```python
from build123d import *

# Parameters (mm, degrees)
SKETCH_R        = 1.75
PAD_DEPTH       = 2
PAD001_DEPTH    = 13
SKETCH002_W     = 76.2
SKETCH002_H     = 61.2
PAD002_DEPTH    = 2
PAD003_DEPTH    = 25
SKETCH004_W     = 14.2
SKETCH004_H     = 19
SKETCH004_W_2   = 29
POCKET_DEPTH    = 2
SKETCH005_W     = 66.2
SKETCH005_H     = 19
POCKET001_DEPTH = 2
SKETCH006_W     = 35
SKETCH006_H     = 25
SKETCH006_W_2   = 14.2
SKETCH006_H_2   = 19
POCKET002_DEPTH = 2
PAD004_DEPTH    = 2
PAD005_DEPTH    = 26
SKETCH009_W     = 51.2
SKETCH009_H     = 20
POCKET003_DEPTH = 2
SKETCH010_W     = 66.2
SKETCH010_H     = 20
POCKET004_DEPTH = 2
SKETCH011_W     = 51.2
SKETCH011_H     = 20
POCKET005_DEPTH = 2
PAD006_DEPTH    = 2
SKETCH013_W     = 5
SKETCH013_H     = 3
PAD007_DEPTH    = 2
SKETCH014_W     = 6
SKETCH014_H     = 6
SKETCH014_R     = 1.25
PAD008_DEPTH    = 6
SKETCH015_W     = 8
SKETCH015_H     = 20
POCKET006_DEPTH = 5
SKETCH016_W     = 20
SKETCH016_H     = 24
POCKET007_DEPTH = 5


with BuildPart() as part:
    # Sketch → Pad (new body)
    with BuildSketch(Plane.XY):
        Polygon((0, 28.537386), (-24.714102, -14.268693), (24.714102, -14.268693), align=None)
        with Locations((7.160898, 4.134347)):
            Circle(SKETCH_R, mode=Mode.SUBTRACT)
        with Locations((0, -8.268693)):
            Circle(SKETCH_R, mode=Mode.SUBTRACT)
        with Locations((-7.160898, 4.134347)):
            Circle(SKETCH_R, mode=Mode.SUBTRACT)
        Polygon((0, 8.537386), (-7.393594, -4.268693), (7.393594, -4.268693), align=None, mode=Mode.SUBTRACT)
    extrude(amount=PAD_DEPTH)

    # Sketch001 (on Face11 of Pad) → Pad001 (join)
    with BuildSketch(Plane.XY.offset(2)):
        Polygon((0, 28.537386), (-24.714102, -14.268693), (24.714102, -14.268693), align=None)
        Polygon((0, 24.537386), (-21.25, -12.268693), (21.25, -12.268693), align=None, mode=Mode.SUBTRACT)
    extrude(amount=PAD001_DEPTH)

    # Sketch002 (on Face14 of Pad001) → Pad002 (join)
    with BuildSketch(Plane.XY.offset(15)):
        with Locations((0, 1.4)):
            Rectangle(SKETCH002_W, SKETCH002_H)
        Polygon((0, 24.537386), (-21.25, -12.268693), (21.25, -12.268693), align=None, mode=Mode.SUBTRACT)
    extrude(amount=PAD002_DEPTH)

    # Sketch003 (on Face23 of Pad002) → Pad003 (join)
    with BuildSketch(Plane.XY.offset(17)):
        Polygon((-38.1, -29.2), (-38.1, 32), (38.1, 32), (38.1, -29.2), (36.1, -29.2), (36.1, -7), (28.1, -7), (28.1, -5), (36.1, -5), (36.1, 30), (-36.1, 30), (-36.1, -5), (-28.1, -5), (-28.1, -7), (-36.1, -7), (-36.1, -29.2), align=None)
    extrude(amount=PAD003_DEPTH)

    # Sketch004 (on Face39 of Pad003) → Pocket (cut)
    with BuildSketch(Plane.YZ.offset(-36.1)):
        with Locations((-17.1, 29.5)):
            Rectangle(SKETCH004_W, SKETCH004_H)
        with Locations((12.5, 29.5)):
            Rectangle(SKETCH004_W_2, SKETCH004_H)
    extrude(amount=-POCKET_DEPTH, mode=Mode.SUBTRACT)

    # Sketch005 (on Face46 of Pocket) → Pocket001 (cut)
    with BuildSketch(Plane.XZ.offset(-30)):
        with Locations((0, 29.5)):
            Rectangle(SKETCH005_W, SKETCH005_H)
    extrude(amount=-POCKET001_DEPTH, mode=Mode.SUBTRACT)

    # Sketch006 (on Face49 of Pocket001) → Pocket002 (cut)
    with BuildSketch(Plane(origin=(36.1, 0, 0), x_dir=(0, -1, 0), z_dir=(-1, 0, 0))):
        with Locations((-12.5, 29.5)):
            Rectangle(SKETCH006_W, SKETCH006_H)
        with Locations((17.1, 29.5)):
            Rectangle(SKETCH006_W_2, SKETCH006_H_2)
    extrude(amount=-POCKET002_DEPTH, mode=Mode.SUBTRACT)

    # Sketch007 (on Face34 of Pocket002) → Pad004 (join)
    with BuildSketch(Plane.XY.offset(42)):
        Polygon((-38.1, -29.2), (-38.1, 32), (38.1, 32), (38.1, -29.2), (28.1, -29.2), (28.1, 22), (-28.1, 22), (-28.1, -29.2), align=None)
    extrude(amount=PAD004_DEPTH)

    # Sketch008 (on Face67 of Pad004) → Pad005 (join)
    with BuildSketch(Plane.XY.offset(44)):
        Polygon((-38.1, -29.2), (-38.1, 32), (38.1, 32), (38.1, -29.2), (36.1, -29.2), (36.1, 30), (-36.1, 30), (-36.1, -29.2), align=None)
    extrude(amount=PAD005_DEPTH)

    # Sketch009 (on Face82 of Pad005) → Pocket003 (cut)
    with BuildSketch(Plane.YZ.offset(-36.1)):
        with Locations((1.4, 57)):
            Rectangle(SKETCH009_W, SKETCH009_H)
    extrude(amount=-POCKET003_DEPTH, mode=Mode.SUBTRACT)

    # Sketch010 (on Face85 of Pocket003) → Pocket004 (cut)
    with BuildSketch(Plane.XZ.offset(-30)):
        with Locations((0, 57)):
            Rectangle(SKETCH010_W, SKETCH010_H)
    extrude(amount=-POCKET004_DEPTH, mode=Mode.SUBTRACT)

    # Sketch011 (on Face88 of Pocket004) → Pocket005 (cut)
    with BuildSketch(Plane(origin=(36.1, 0, 0), x_dir=(0, -1, 0), z_dir=(-1, 0, 0))):
        with Locations((-1.4, 57)):
            Rectangle(SKETCH011_W, SKETCH011_H)
    extrude(amount=-POCKET005_DEPTH, mode=Mode.SUBTRACT)

    # Sketch012 (on Face78 of Pocket005) → Pad006 (join)
    with BuildSketch(Plane.XY.offset(70)):
        Polygon((-38.1, -29.2), (-38.1, 32), (38.1, 32), (38.1, -29.2), (31.1, -29.2), (31.1, -25.2), (34.1, -25.2), (34.1, 28), (-34.1, 28), (-34.1, -25.2), (-31.1, -25.2), (-31.1, -29.2), align=None)
    extrude(amount=PAD006_DEPTH)

    # Sketch013 (on Face98 of Pad006) → Pad007 (join)
    with BuildSketch(Plane.XZ.offset(29.2)):
        with Locations((-33.6, 68.5)):
            Rectangle(SKETCH013_W, SKETCH013_H)
        with Locations((33.6, 68.5)):
            Rectangle(SKETCH013_W, SKETCH013_H)
    extrude(amount=-PAD007_DEPTH)

    # Sketch014 (on Face19 of Pad007) → Pad008 (join)
    with BuildSketch(Plane.XZ.offset(29.2)):
        with Locations((31.1, 12)):
            Rectangle(SKETCH014_W, SKETCH014_H)
        with Locations((31.1, 12)):
            Circle(SKETCH014_R, mode=Mode.SUBTRACT)
        with Locations((-8.9, 12)):
            Rectangle(SKETCH014_W, SKETCH014_H)
        with Locations((-8.9, 12)):
            Circle(SKETCH014_R, mode=Mode.SUBTRACT)
    extrude(amount=-PAD008_DEPTH)

    # Sketch015 (on Face83 of Pad008) → Pocket006 (cut)
    with BuildSketch(Plane.XY.offset(44)):
        with Locations((-32.1, 5)):
            Rectangle(SKETCH015_W, SKETCH015_H)
    extrude(amount=-POCKET006_DEPTH, mode=Mode.SUBTRACT)

    # Sketch016 (on Face61 of Pocket006) → Pocket007 (cut)
    with BuildSketch(Plane.YZ.offset(-36.1)):
        with Locations((5, 32)):
            Rectangle(SKETCH016_W, SKETCH016_H)
    extrude(amount=-POCKET007_DEPTH, mode=Mode.SUBTRACT)


solid = part.part
```
Part model, mm, in its own coordinate system. A direction names the side the tool comes from. Round coordinates to 2 decimals unless told otherwise and drop trailing zeros. Loops run counter-clockwise (first coordinate to the right, second up) from the corner with the lowest first, then second, coordinate; pieces in that order, holes last.
1. Slice it at A-A (z = 12). Give the cut face in (x, y).
Solutions:
outline: (-24.71, -14.27) - (24.71, -14.27) - (0, 28.54) - close; (-11.9, -29.2) - (-10.15, -29.2) - (-10.15, -23.2) - (-11.9, -23.2) - close; (-7.65, -29.2) - (-5.9, -29.2) - (-5.9, -23.2) - (-7.65, -23.2) - close; (28.1, -29.2) - (29.85, -29.2) - (29.85, -23.2) - (28.1, -23.2) - close; (32.35, -29.2) - (34.1, -29.2) - (34.1, -23.2) - (32.35, -23.2) - close; hole (-21.25, -12.27) - (21.25, -12.27) - (0, 24.54) - close
2. Slice it at B-B (x = 4). Count the separate pieces of the cut face and the enclosed holes in it, and give its area (3 significant figures).
Solutions:
separate pieces: 4
enclosed holes: 0
area: 253 mm2
3. Slice it at C-C (z = 52). Give the cut face in (x, y).
Solutions:
outline: (-38.1, -29.2) - (-36.1, -29.2) - (-36.1, -24.2) - (-38.1, -24.2) - close; (-38.1, 27) - (-36.1, 27) - (-36.1, 30) - (-33.1, 30) - (-33.1, 32) - (-38.1, 32) - close; (33.1, 30) - (36.1, 30) - (36.1, 27) - (38.1, 27) - (38.1, 32) - (33.1, 32) - close; (36.1, -29.2) - (38.1, -29.2) - (38.1, -24.2) - (36.1, -24.2) - close
4. Two-plate mould, pull along Y, no slides. Class faces 6 (the face through (33.1, 31, 29)), 7 (the face through (0, 29, 70)): pulls with the +Y half, pulls with the -Y half, needs draft (parallel to the pull), parting line crosses it, or undercut.
Solutions:
face 6: needs draft
face 7: undercut
5. 3-axis set-ups, long thin cutter, end or side, ignore diameter. For faces 1 (the face through (-37, -24.2, 57)), 2 (the face through (0, -12.269, 9)), 3 (the face through (-28.1, -6, 36)), 4 (the face through (-10.3, -23.2, 12)), 5 (the face through (-36.1, 18, 19)): which of +Z, -Z, +X, -X, +Y, -Y reach the whole face in a straight line?
Solutions:
face 1: +X, -X
face 2: +Z
face 3: +Z, -Y
face 4: -Z, +X, -X
face 5: +X
6. Flat gauge pins, fed straight in: pin 1 (6.5 mm diameter, centred on x = -30, z = 33, fed in from -Y); pin 2 (6.5 mm diameter, centred on x = -8, y = -27.5, fed in from -Z); pin 3 (1 mm diameter, centred on x = -14.5, z = 12, fed in from +Y). Where does each tip first touch, or does it go through?
Solutions:
pin 1: stops at y = -7
pin 2: stops at z = 9
pin 3: stops at y = 4.29
7. Drill centre lines: line 1 along Z through (x, y) = (31, -25); line 2 along Z through (x, y) = (33.5, 11); line 3 along Z through (x, y) = (-32, -0.5). Where is each one in solid material? Low to high.
Solutions:
line 1: z = 9 to 10.75, 13.25 to 17, 42 to 44
line 2: z = 15 to 17, 42 to 44
line 3: z = 15 to 17
8. Slice it at D-D (x = 16). Give the cut face in (y, z), and give its area (3 significant figures).
Solutions:
outline: (-29.2, 15) - (-14.27, 15) - (-14.27, 0) - (0.82, 0) - (0.82, 15) - (32, 15) - (32, 20) - (30, 20) - (30, 17) - (-3.18, 17) - (-3.18, 2) - (-12.27, 2) - (-12.27, 17) - (-29.2, 17) - close; (22, 42) - (30, 42) - (30, 39) - (32, 39) - (32, 47) - (30, 47) - (30, 44) - (22, 44) - close; (28, 70) - (30, 70) - (30, 67) - (32, 67) - (32, 72) - (28, 72) - close
area: 264 mm2
